```python
from build123d import *

# Parameters (mm, degrees)
F3_R     = 2.6577794355
F4_DEPTH = 45
F5_SIZE2 = 0.6984153898
F5_SIZE  = 20


# Not quite as in the source:
# - a fillet or chamfer that OpenCascade refuses, or shapes differently, is made with other operations: its cross-section is extruded or revolved along the edge and cut away or added


with BuildPart() as f1:
    # F0 (on Top) → F1 (revolve)
    with BuildSketch(Plane.XY):
        Polygon((25, 21.8126288628), (1.5, 21.8126288628), (1.5, -2.4768179283), (15.309067443, -2.4768179283), (15.9076526761, -3.1873711372), (16.5, -3.1873711372), (16.5, -0.1873711372), (9.0524229015, 0), (9.0524229015, 19.8126288628), (25, 19.8126288628), align=None)
    revolve(axis=Axis((0, 9.3126288628, 0), (0, 1, 0)))

    # F2: fillet of radius 1 on 2 edges, made by hand

    # F2_s1 → F2_t2 (revolve, cut)
    with BuildSketch(Plane.XY):
        with BuildLine():
            ThreePointArc((15.9076526761, -3.1873711372), (16.3389435845, -2.8184524698), (16.5, -2.2742340743))
            Line((16.5, -2.2742340743), (16.5, -3.1873711372))
            Line((16.5, -3.1873711372), (15.9076526761, -3.1873711372))
        make_face()
    revolve(axis=Axis((0, -3.1873711372, 0), (0, 1, 0)), mode=Mode.SUBTRACT)

    # F2_s3 → F2_t4 (revolve, cut)
    with BuildSketch(Plane.XY):
        with BuildLine():
            ThreePointArc((16.5, -1.1625288961), (16.2159436821, -0.4643708596), (15.5251507119, -0.1628452253))
            Line((15.5251507119, -0.1628452253), (16.5, -0.1873711372))
            Line((16.5, -0.1873711372), (16.5, -1.1625288961))
        make_face()
    revolve(axis=Axis((0, -0.1873711372, 0), (0, 1, 0)), mode=Mode.SUBTRACT)

    # F3 (on Top) → F4 (join)
    with BuildSketch(Plane.XY):
        with Locations((0, 10.5296224356)):
            Circle(F3_R)
    extrude(amount=F4_DEPTH)

    # F5
    f5_edges = [f1.edges().sort_by_distance(p)[0] for p in [
        (-2.657779, 10.529622, 45),
    ]]
    f5_side = f1.faces().sort_by_distance((-2.657779, 10.529622, 26.826736))[0]
    chamfer(f5_edges, length=F5_SIZE, length2=F5_SIZE2, reference=f5_side)


solid = f1.part
```
Design review of the part built by this model. Coordinates are the model's own, in mm. A direction names the side the tool comes from. Coordinates: 2 decimals unless noted, no trailing zeros. Write each loop counter-clockwise with the first axis right and the second up, starting at its lowest first coordinate (ties: lowest second). Pieces come first, ordered by that corner, then holes.
1) Insertion check: pin 1 (2.5 mm diameter, centred on x = 0, z = 0, fed in from +Y); pin 2 (5 mm diameter, centred on x = 0.5, y = 3, fed in from -Z); pin 3 (1.5 mm diameter, centred on y = 9.5, z = -2, fed in from +X). Each pin has a flat end and moves straight along its axis. Give the tip position at first contact, or say it passes through.
2) Mouldability with a two-part tool opening along Z and no side actions: class faces 5 (the flat face through (0, 11, 0)), 6 (the cylindrical face through (-1.178, 10.045, -8.975)), 7 (the conical face through (2.197, 11.222, 35.14)) as +Z half, -Z half, draft (parallel to the pull), parting line (faces both ways), or undercut.
3) Add section B-B (y = 17.75). Write out the cut boundary in (x, z).
4) Add section D-D (x = 21). Write out the cut boundary in (y, z).
5) Machinability: for faces 1 (the flat face through (0, -2.477, 3)), 2 (the cylindrical face through (1.226, 8.172, 16.712)), 3 (the flat face through (0, 11, 45)), 4 (the conical face through (8.934, -0.008, -2.814)), which of the approach directions +Z, -Z, +X, -X, +Y, -Y give a long, thin tool a straight path to every point of the face, cutting with its end or side? Answer none if there is none.
6) To check wall thickness, follow L1, parallel to X at y = 5.5, z = 0; L2, parallel to Y at x = 16.5, z = 14. State the ranges of each line that lie inside material, in increasing order.
7) Add section C-C (z = 33). Write out the cut boundary in (x, y), plus the area to 3 significant figures.
Check result:
1. pin 1: stops at y = 13.19
1. pin 2: stops at z = -9.05
1. pin 3: stops at x = 8.97
2. face 5: undercut
2. face 6: parting line
2. face 7: +Z half
3. outline: circle Ø18.1 at (0, 0); hole circle Ø3 at (0, 0)
4. outline: (19.81, -13.56) - (21.81, -13.56) - (21.81, 13.56) - (19.81, 13.56) - close
5. face 1: -Y
5. face 2: +Z
5. face 3: +Z, +X, -X, +Y, -Y
5. face 4: none
6. L1: x = -9.05 to -1.5, 1.5 to 9.05
6. L2: y = 19.81 to 21.81
7. outline: circle Ø4.76 at (0, 10.53)
7. area: 17.8 mm2
